```python
from build123d import *

# Parameters (mm, degrees)
BOSS_EXTRUDE1_DEPTH = 145
SKETCH2_W           = 68.65
SKETCH2_H           = 145
CUT_EXTRUDE1_DEPTH  = 10
SKETCH3_R           = 7
CUT_EXTRUDE2_DEPTH  = 10
SKETCH4_R           = 2.55
CUT_EXTRUDE3_DEPTH  = 10
SKETCH5_W           = 278.618693002
SKETCH5_H           = 61.467749786
CUT_EXTRUDE4_DEPTH  = 10


with BuildPart() as part:
    # Sketch1 → Boss-Extrude1 (new body)
    with BuildSketch(Plane.XY):
        Polygon((0, -37.5), (0, 37.5), (75, 37.5), (75, 31.15), (6.35, 31.15), (6.35, -31.15), (75, -31.15), (75, -37.5), align=None)
    extrude(amount=BOSS_EXTRUDE1_DEPTH)

    # Sketch2 → Cut-Extrude1 (cut)
    with BuildSketch(Plane(origin=(0, 37.5, 0), x_dir=(1, 0, 0), z_dir=(0, 1, 0))):
        with Locations((40.675, -72.5)):
            Rectangle(SKETCH2_W, SKETCH2_H)
    extrude(amount=-CUT_EXTRUDE1_DEPTH, mode=Mode.SUBTRACT)

    # Sketch3 → Cut-Extrude2 (cut)
    with BuildSketch(Plane.XZ.offset(37.5)):
        with Locations(Location((40, 72.5, 0), (0, 0, 270))):
            Circle(SKETCH3_R)
    extrude(amount=-CUT_EXTRUDE2_DEPTH, mode=Mode.SUBTRACT)

    # Sketch4 → Cut-Extrude3 (cut)
    with BuildSketch(Plane(origin=(0, -31.15, 0), x_dir=(1, 0, 0), z_dir=(0, 1, 0))):
        with Locations(Location((59.798989873, -52.701010127, 0), (0, 0, 270))):
            Circle(SKETCH4_R)
        with Locations(Location((59.798989873, -92.298989873, 0), (0, 0, 270))):
            Circle(SKETCH4_R)
        with Locations(Location((20.201010127, -92.298989873, 0), (0, 0, 270))):
            Circle(SKETCH4_R)
        with Locations(Location((20.201010127, -52.701010127, 0), (0, 0, 270))):
            Circle(SKETCH4_R)
    extrude(amount=-CUT_EXTRUDE3_DEPTH, mode=Mode.SUBTRACT)

    # Sketch5 → Cut-Extrude4 (cut)
    with BuildSketch(Plane(origin=(6.35, 0, 0), x_dir=(0, 0, -1), z_dir=(1, 0, 0))):
        with Locations((-29.250225685, 27.958406515)):
            Rectangle(SKETCH5_W, SKETCH5_H)
    extrude(amount=-CUT_EXTRUDE4_DEPTH, mode=Mode.SUBTRACT)


solid = part.part
```
Could you check a few things on this model? Use its own coordinates, in mm. A direction names the side the tool comes from. Round coordinates to 2 decimals unless told otherwise and drop trailing zeros. Loops run counter-clockwise (first coordinate to the right, second up) from the corner with the lowest first, then second, coordinate; pieces in that order, holes last. Notation, with made-up numbers: (10.5, 11) - (14.5, 11) arc R28 cw to (14.5, 40) - close; hole circle Ø9 at (4.5, -20). An arc over 180 degrees is marked (long way). Use CSV: the item, a comma, the result in double quotes.
Item 1: If we section it at C-C on z = 98: List the corners of the cut face in (x, y) for me, then the cut area to 3 significant figures.
Here are the results:
outline,"(0, -37.5) - (75, -37.5) - (75, -31.15) - (6.35, -31.15) - (6.35, -2.78) - (0, -2.78) - close"
area,"656 mm²"
Item 2: Will these pins go through, and if not, where does the flat tip stop? pin 1 (6.5 mm diameter, centred on x = 59.8, z = 92.3, fed in from -Y); pin 2 (2 mm diameter, centred on x = 53.5, z = 58.5, fed in from +Y).
Here are the results:
pin 1,"stops at y = -37.5"
pin 2,"stops at y = -31.15"
Item 3: For faces 1 (the flat face through (0, -20, 71)), 2 (the flat face through (33, -31.15, 71)), which set-ups out of +Z, -Z, +X, -X, +Y, -Y let a thin tool reach every point of the face, with its end or its side?
Here are the results:
face 1,"+Z, -Z, -X, +Y, -Y"
face 2,"+Z, -Z, +X, +Y"
Item 4: If we mould it in two halves opening along X, with no side actions, what happens to faces 3 (the cylindrical face through (20.967, -34.281, 55.133)), 4 (the flat face through (6.35, -17, 74)), 5 (the flat face through (29, -32, 0))? For each: pulls with the +X half, pulls with the -X half, needs draft (parallel to the pull), parting line crosses it, or undercut.
Here are the results:
face 3,"undercut"
face 4,"pulls with the +X half"
face 5,"needs draft"
Item 5: If we section it at B-B on z = 72.5: List the corners of the cut face in (x, y) for me, then the cut area to 3 significant figures.
Here are the results:
outline,"(0, -37.5) - (33, -37.5) - (33, -31.15) - (6.35, -31.15) - (6.35, -2.78) - (0, -2.78) - close; (47, -37.5) - (75, -37.5) - (75, -31.15) - (47, -31.15) - close"
area,"568 mm²"
Item 6: If we section it at D-D on y = -33.5: List the corners of the cut face in (x, z) for me, then the cut area to 3 significant figures.
Here are the results:
outline,"(0, 0) - (75, 0) - (75, 145) - (0, 145) - close; hole circle Ø5.1 at (20.2, 52.7); hole circle Ø5.1 at (20.2, 92.3); hole circle Ø14 at (40, 72.5); hole circle Ø5.1 at (59.8, 52.7); hole circle Ø5.1 at (59.8, 92.3)"
area,"10,600 mm²"
Item 7: If we section it at A-A on x = 40: List the corners of the cut face in (y, z) for me.
Here are the results:
outline,"(-37.5, 0) - (-31.15, 0) - (-31.15, 65.5) - (-37.5, 65.5) - close; (-37.5, 79.5) - (-31.15, 79.5) - (-31.15, 145) - (-37.5, 145) - close"
Item 8: I need wall thicknesses on L1, parallel to Y at x = 62.5, z = 95.5; L2, parallel to X at y = -24, z = 86. Which ranges of each line are inside material? Lowest first, please. Write a range as [from, to].
Here are the results:
L1,"y = [-37.5, -31.15]"
L2,"x = [0, 6.35]"
